Autodesk Inventor part; units mm, degrees
ref_plane "Plano inicial" through (0, 0, -25.4) normal (0, 0, 1) x (1, 0, 0)
ref_plane "Plano final" through (0, 0, 230) normal (0, 0, 1) x (1, 0, 0)
ref_plane "Plano de trabajo4" through (-25.4, 0, -25.4) normal (0.7071, 0, -0.7071) x (-0.7071, 0, -0.7071)
ref_plane "Plano inicial" through (0, 0, -25.4) normal (0, 0, 1) x (1, 0, 0)
ref_plane "Plano final" through (0, 0, 230) normal (0, 0, 1) x (1, 0, 0)
sketch "Boceto" plane through (0, 0, 0) normal (0, 0, 1) x (1, 0, 0)
  line L0 (-25.4, -19.05) -> (-25.4, 19.05)
  line L1 (-19.05, 25.4) -> (19.05, 25.4)
  line L2 (25.4, 19.05) -> (25.4, -19.05)
  line L3 (19.05, -25.4) -> (-19.05, -25.4)
  arc A0 (-25.4, -19.05) -> (-19.05, -25.4) centre (-19.05, -19.05) ccw
  arc A1 (-19.05, 25.4) -> (-25.4, 19.05) centre (-19.05, 19.05) ccw
  arc A2 (25.4, 19.05) -> (19.05, 25.4) centre (19.05, 19.05) ccw
  arc A3 (19.05, -25.4) -> (25.4, -19.05) centre (19.05, -19.05) ccw
  arc A4 (-19.05, 22.225) -> (-22.225, 19.05) centre (-19.05, 19.05) ccw
  line L4 (-19.05, 22.225) -> (19.05, 22.225)
  arc A5 (22.225, 19.05) -> (19.05, 22.225) centre (19.05, 19.05) ccw
  line L5 (22.225, 19.05) -> (22.225, -19.05)
  arc A6 (19.05, -22.225) -> (22.225, -19.05) centre (19.05, -19.05) ccw
  line L6 (19.05, -22.225) -> (-19.05, -22.225)
  arc A7 (-22.225, -19.05) -> (-19.05, -22.225) centre (-19.05, -19.05) ccw
  line L7 (-22.225, -19.05) -> (-22.225, 19.05)
  line L8 (0, 37.4012) -> (0, -37.4012) construction
  line L9 (-37.4012, 0) -> (37.4012, 0) construction
  dimension "d10" = 50.8
  dimension "d11" = 50.8
  dimension "d12" = 3.175
  dimension "d15" = 25.4
  dimension "d16" = 25.4
  dimension "d17" = 6.35
extrude "Cuerpo" add sketch "Boceto" along normal up to surface (255.4 mm away) from surface at -25.4
sketch "Sketch3" plane through (0, 0, 0) normal (0, 0, 1) x (1, 0, 0)
  line L0 (0, 0) -> (10, 0)
ref_plane "Work Plane3" through (0, 0, 0) normal (0, -1, 0) x (1, 0, 0)
ref_plane "Plano de trabajo4" through (-25.4, 0, -25.4) normal (0.7071, 0, -0.7071) x (-0.7071, 0, -0.7071)
split "Dividir1" plane through (-25.4, 0, -25.4) removes the side toward (0.7071, 0, -0.7071)
sketch "Sketch4" plane through (0, 0, 0) normal (0, -1, 0) x (1, 0, 0)
  line L0 (-2, -25.4) -> (12, -25.4)
  line L1 (-2, 230) -> (12, 230)
  dimension "d19" = 255.4
equation "\"d10\" = G_H"
equation "\"d11\" = G_W"
equation "\"d12\" = G_T"
equation "\"d15\" = 0.5 * d10"
equation "\"d16\" = 0.5 * d11"
equation "\"d17\" = G_IR"
equation "\"d3\" = G_L"
equation "\"G_W\" = 50.8"
equation "\"G_H\" = 50.8"
equation "\"G_T\" = 3.175"
equation "\"G_IR\" = 6.35"
equation "\"G_L\" = d19"
equation "\"G_OFFSET_START\" = 25.4"
equation "\"G_OFFSET_END\" = 0"
equation "\"d13\" = -G_OFFSET_START"
properties part number "AISC - 2 x 2 x 1/8 - 10,055" material "Acero, suave"
Geometry check sheet. Reference: the model listing, model coordinates, mm. A direction names the side the tool comes from. Round coordinates to 2 decimals unless told otherwise and drop trailing zeros. Order: outer loops, then holes, each group sorted by start corner. A loop starts at its lowest first (then second) coordinate and runs counter-clockwise, first axis right, second up. Notation, with made-up numbers: M 34,-18 L 76,-18 A22 ccw 76,15 Z; hole C 16.25,53.25 d2. An arc over 180 degrees is marked long. Answer in a Markdown table with one row per item. Add a question column.
Item 1: Set-up check for faces 1 (the face through (-25.4, 0, 101)), 2 (the face through (0, 22.225, 104)): record each of +Z, -Z, +X, -X, +Y, -Y from which the full face is reachable in a straight line by a thin tool's end or side.
Item 2: Sectioned sample at D-D, the plane z = 12.5. Enter the section's corners in (x, y) (3 decimals).
Item 3: Sectioned sample at B-B, the plane y = -13. Enter the section's corners in (x, z) (3 decimals).
Item 4: Material ranges on L1, parallel to Y at x = 0, z = 205.5 (3 decimals); L2, parallel to X at y = -18, z = -10 (3 decimals), recorded low to high. Write a range as [from, to].
Item 5: Draft check along Y on faces 3 (the face through (-23.59, 23.49, 100.51)), 4 (the face through (-0.1, -22.5, 230)), 5 (the face through (22.225, 0, 125)), 6 (the face through (-22.225, 0, 102)). Enter one of: released by +Y, released by -Y, zero draft, split by the parting line, or undercut.
Item 6: Depth check by flat-ended pin: pin 1 Ø10 at (x, y) = (14.5, 19) entering from +Z. Enter the tip coordinate at first touch or a pass-through.
Item 7: Sectioned sample at C-C, the plane z = 204.5. Enter the section's corners in (x, y) (3 decimals).
Item 8: Sectioned sample at A-A, the plane x = -7. Enter the section's corners in (y, z) (3 decimals), plus the area to 3 significant figures.
Filled in:
| question | item | result |
|---|---|---|
| 1 | face 1 | +Z, -Z, -X, +Y, -Y |
| 1 | face 2 | +Z, -Z |
| 2 | outline | M -25.4,-19.05 A6.35 ccw -19.05,-25.4 L 12.5,-25.4 L 12.5,-22.225 L -19.05,-22.225 A3.175 cw -22.225,-19.05 L -22.225,19.05 A3.175 cw -19.05,22.225 L 12.5,22.225 L 12.5,25.4 L -19.05,25.4 A6.35 ccw -25.4,19.05 Z |
| 3 | outline | M -25.4,-25.4 L -22.225,-22.225 L -22.225,230 L -25.4,230 Z; M 22.225,22.225 L 25.4,25.4 L 25.4,230 L 22.225,230 Z |
| 4 | L1 | y = [-25.4, -22.225], [22.225, 25.4] |
| 4 | L2 | x = [-25.4, -22.225] |
| 5 | face 3 | released by +Y |
| 5 | face 4 | zero draft |
| 5 | face 5 | undercut |
| 5 | face 6 | undercut |
| 6 | pin 1 | stops at z = 230 |
| 7 | outline | M -25.4,-19.05 A6.35 ccw -19.05,-25.4 L 19.05,-25.4 A6.35 ccw 25.4,-19.05 L 25.4,19.05 A6.35 ccw 19.05,25.4 L -19.05,25.4 A6.35 ccw -25.4,19.05 Z; hole M -22.225,-19.05 A3.175 ccw -19.05,-22.225 L 19.05,-22.225 A3.175 ccw 22.225,-19.05 L 22.225,19.05 A3.175 ccw 19.05,22.225 L -19.05,22.225 A3.175 ccw -22.225,19.05 Z |
| 8 | outline | M -25.4,-7 L -22.225,-7 L -22.225,230 L -25.4,230 Z; M 22.225,-7 L 25.4,-7 L 25.4,230 L 22.225,230 Z |
| 8 | area | 1,500 mm² |
